Input: part model. Units: mm. Frame: model coordinates. A direction names the side the tool comes from. Coordinates: 2 decimals unless noted, no trailing zeros. Loops run counter-clockwise (first coordinate to the right, second up) from the corner with the lowest first, then second, coordinate; pieces in that order, holes last. Notation, with made-up numbers: (-7, 16.5) - (14, 16.5) arc R11 ccw to (14, 29.5) - close; hole circle Ø8 at (82.25, 83.25). An arc over 180 degrees is marked (long way). Write item = value, one per line. Start each with the question number.
from build123d import *

# Parameters (mm, degrees)
SKETCH2_R          = 1.5875
CUT_EXTRUDE1_DEPTH = 6.35


with BuildPart() as part:
    # Sketch1 → Revolve1 (revolve)
    with BuildSketch(Plane(origin=(0, 0, 0), x_dir=(0, 0, -1), z_dir=(1, 0, 0)), mode=Mode.PRIVATE) as revolve1_sk:
        Polygon((0, 0), (0, 36.261189321), (0, 67.945), (4.064, 67.945), (4.064, 61.0235), (1.5875, 61.0235), (1.5875, 58.42), (4.94665, 58.42), (4.94665, 55.0418), (14.42085, 55.0418), (14.42085, 49.8348), (15.08125, 49.8348), (15.08125, 15.7734), (14.42085, 15.7734), (14.42085, 7.9756), (4.9911, 7.9756), (4.9911, 5.4102), (1.5748, 5.4102), (1.5748, 0), align=None)
    revolve(revolve1_sk.sketch.rotate(Axis((0, 67.945, 0), (0, -1, 0)), 180), axis=Axis((0, 67.945, 0), (0, -1, 0)))

    # Sketch2 → Cut-Extrude1 (cut)
    with BuildSketch(Plane(origin=(0, 55.0418, 0), x_dir=(1, 0, 0), z_dir=(0, 1, 0))):
        with Locations(Location((-10.414, 0, 0), (0, 0, 270))):
            Circle(SKETCH2_R)
        with Locations(Location((10.414, 0, 0), (0, 0, 90))):
            Circle(SKETCH2_R)
    extrude(amount=-CUT_EXTRUDE1_DEPTH, mode=Mode.SUBTRACT)


solid = part.part
Item 1: Cut plane A-A on z = 9. Return loops of the section in (x, y).
Item 2: Cut plane C-C on y = 38.5. Return loops of the section in (x, z).
Item 3: Pin query (flat end, axial travel): pin 1 (12 mm diameter, centred on x = -11.5, y = 38.5, fed in from -Z); pin 2 (4 mm diameter, centred on x = -10.414, z = 0, fed in from +Y); pin 3 (2 mm diameter, centred on x = 3.5, y = 19.5, fed in from -Z). Return the tip coordinate at first contact, or that it passes through.
Item 4: Access query for faces 4 (the cylindrical face through (-8.84, 51.91, -0.21)), 5 (the flat face through (0, 7.976, 6)), 6 (the cylindrical face through (1.41, 59.7, 0.73)), 7 (the flat face through (0, 0, 0)). Directions: +Z, -Z, +X, -X, +Y, -Y. A direction counts if a zero-diameter tool reaches every point of the face in a straight line with its end or side. Return the directions, or none.
Item 5: Cut plane D-D on y = 51. Return loops of the section in (x, z) (1 decimal), plus the area to 3 significant figures.
Item 6: Pull-direction query (Z, two-part tool) for faces 1 (the flat face through (10, 48.692, 0)), 2 (the cylindrical face through (0.96, 2.67, -1.25)), 3 (the flat face through (0, 67.945, 0)); classes: pulls with the +Z half, pulls with the -Z half, needs draft (parallel to the pull), parting line crosses it, or undercut.
Item 7: Ray query, line 1 (X direction, y = 53, z = 0); line 2 (Y direction, x = 1, z = 3.5) (1 decimal); line 3 (X direction, y = 53, z = 0.5). Return the intervals inside material, ascending.
Recorded:
q1.outline = (-12.1, 15.77) - (-11.27, 15.77) - (-11.27, 7.98) - (11.27, 7.98) - (11.27, 15.77) - (12.1, 15.77) - (12.1, 49.83) - (11.27, 49.83) - (11.27, 55.04) - (-11.27, 55.04) - (-11.27, 49.83) - (-12.1, 49.83) - close
q2.outline = circle Ø30.16 at (0, 0)
q3.pin_1 = -14.04
q3.pin_2 = 55.04
q3.pin_3 = -14.87
q4.face_4 = +Y
q4.face_5 = -Y
q4.face_6 = none
q4.face_7 = +Z, -Z, +X, -X, -Y
q5.outline = circle Ø28.8 at (0, 0); hole circle Ø3.2 at (-10.4, 0); hole circle Ø3.2 at (10.4, 0)
q5.area = 637 mm²
q6.face_1 = undercut
q6.face_2 = parting line crosses it
q6.face_3 = needs draft
q7.line_1 = -14.42 to -12, -8.83 to 8.83, 12 to 14.42
q7.line_2 = 5.4 to 58.4, 61 to 67.9
q7.line_3 = -14.41 to -11.92, -8.91 to 8.91, 11.92 to 14.41
